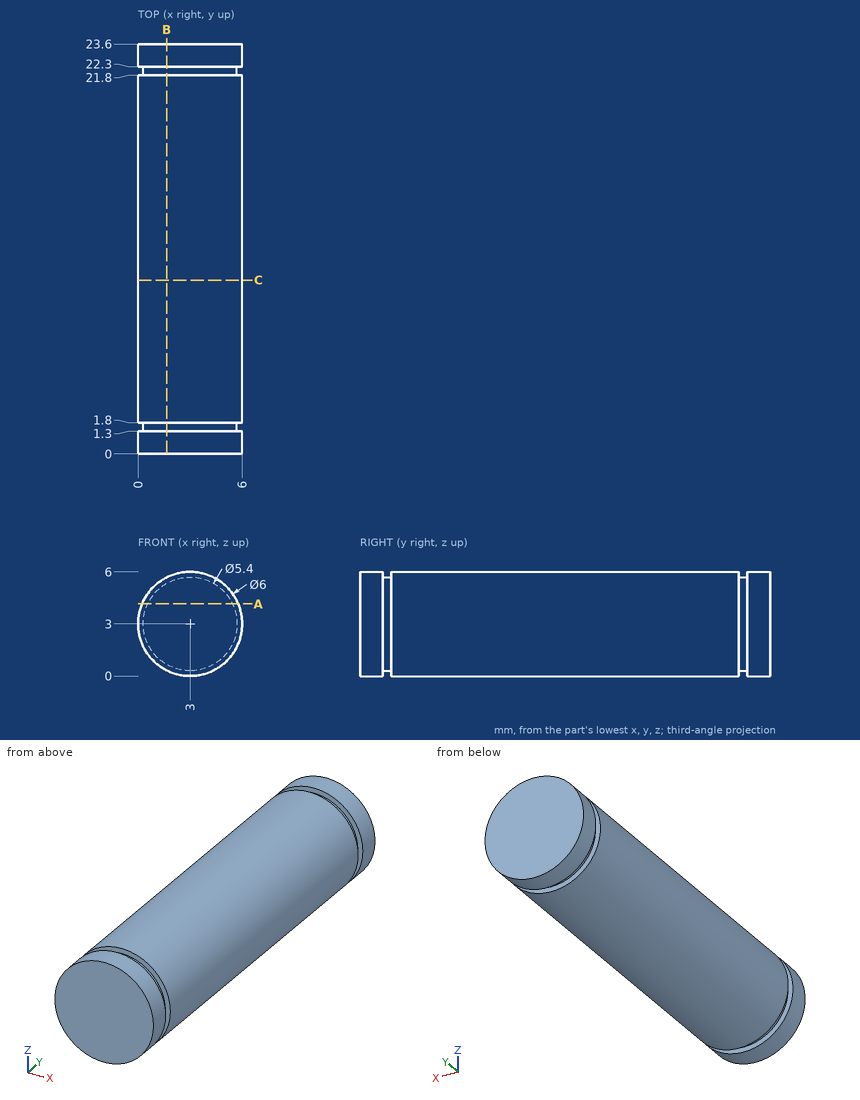
Source: three-view drawing plus pictorial views. Frame: mm from the lowest corner of the part. Coordinates: 2 decimals unless noted, no trailing zeros. Order: outer loops, then holes, each group sorted by start corner. A loop starts at its lowest first (then second) coordinate and runs counter-clockwise, first axis right, second up. Notation, with made-up numbers: M -23,48.5 L 3,48.5 A23 cw 3,81.5 Z; hole C -30,1.25 d1. An arc over 180 degrees is marked long. Write each question's results on one line, items separated by ' | '. Start each with the question number.
1. Material intervals for L1, parallel to Y at x = 4.3, z = 5.6; L2, parallel to Z at x = 0.85, y = 14.5; L3, parallel to X at y = 7.75, z = 0.65, sorted ascending.
2. Pin query (flat end, axial travel): pin 1 (1 mm diameter, centred on x = 5, y = 14, fed in from +Z); pin 2 (1.5 mm diameter, centred on x = 2.5, z = 2, fed in from -Y); pin 3 (1.5 mm diameter, centred on y = 17.5, z = 2, fed in from +X). Return the tip coordinate at first contact, or that it passes through.
3. Section B-B, the plane x = 1.65. Return the cut outline in (y, z).
4. Section C-C, the plane y = 10. Return the cut outline in (x, z).
5. Section A-A, the plane z = 4.15. Return the cut outline in (x, y), then the cut area to 3 significant figures.
Solution:
1) L1: 0 to 1.3, 1.8 to 21.8, 22.3 to 23.6 | L2: 0.91 to 5.09 | L3: 1.14 to 4.86
2) pin 1: z = 5.6 | pin 2: y = 0 | pin 3: x = 5.99
3) outline: M 0,0.32 L 1.3,0.32 L 1.3,0.66 L 1.8,0.66 L 1.8,0.32 L 21.8,0.32 L 21.8,0.66 L 22.3,0.66 L 22.3,0.32 L 23.6,0.32 L 23.6,5.68 L 22.3,5.68 L 22.3,5.34 L 21.8,5.34 L 21.8,5.68 L 1.8,5.68 L 1.8,5.34 L 1.3,5.34 L 1.3,5.68 L 0,5.68 Z
4) outline: C 3,3 d6
5) outline: M 0.23,0 L 5.77,0 L 5.77,1.3 L 5.44,1.3 L 5.44,1.8 L 5.77,1.8 L 5.77,21.8 L 5.44,21.8 L 5.44,22.3 L 5.77,22.3 L 5.77,23.6 L 0.23,23.6 L 0.23,22.3 L 0.56,22.3 L 0.56,21.8 L 0.23,21.8 L 0.23,1.8 L 0.56,1.8 L 0.56,1.3 L 0.23,1.3 Z | area: 130 mm²
